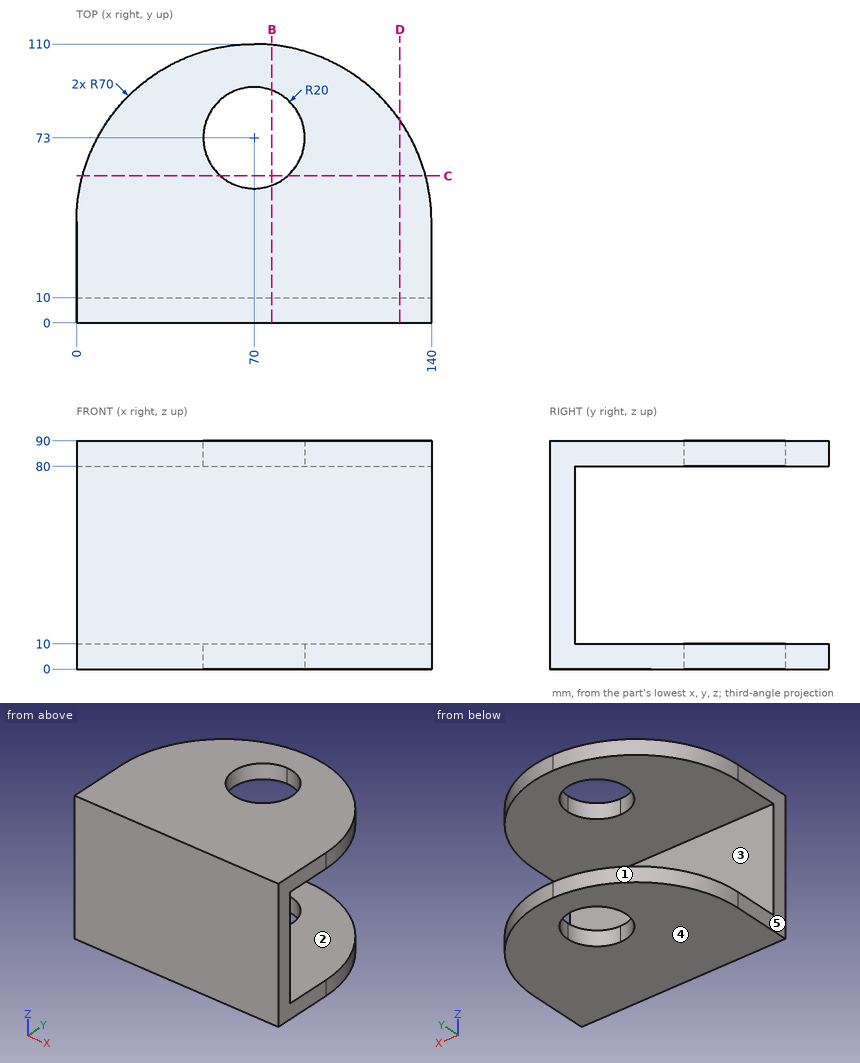
Input: dimensioned drawing with shaded views. Units: mm. Origin: part minimum x, y, z. A direction names the side the tool comes from. Give positions to 0.01 mm unless a question says otherwise; leave off trailing zeros. Loops run counter-clockwise (first coordinate to the right, second up) from the corner with the lowest first, then second, coordinate; pieces in that order, holes last. Notation, with made-up numbers: M -28.75,69.25 L 10.25,69.25 A27 ccw 10.25,97.25 Z; hole C 25,33 d3. An arc over 180 degrees is marked long. Put each result on its own line as item: value.
1) Mould query, pull axis Z, two halves, no side actions, for the marked faces 3, 4 and 5. Classes: released by +Z, released by -Z, zero draft, split by the parting line, or undercut.
Computed values:
face 3: undercut
face 4: released by -Z
face 5: zero draft
2) Reachability of the marked faces 1 and 2 from +Z, -Z, +X, -X, +Y, -Y: full face, straight path, thin tool, end or side. Return the list, or none.
Computed values:
face 1: +Z, -Z, -X, +Y
face 2: +X, -X, +Y
3) First-contact query: P1, Ø12, axis at y = 61, z = 17.5, coming from the -X side; P2, Ø10, axis at x = 104, z = 75.5, coming from the +Y side; P3, Ø21, axis at x = 46, z = 46.5, coming from the +Y side. Flat tips, straight axial feed; report the tip coordinate or a pass-through.
Computed values:
P1: passes through
P2: stops at y = 102.35
P3: stops at y = 10
4) Material intervals for L1, parallel to Z at x = 51.5, y = 60.5; L2, parallel to Y at x = 114, z = 17; L3, parallel to Y at x = 68.5, z = 8, sorted ascending. Write a range as from..to.
Computed values:
L1: z = 0..10, 80..90
L2: y = 0..10
L3: y = 0..53.06, 92.94..109.98
5) Cut plane B-B, the plane x = 77. Return the cut outline in (y, z) (3 decimals).
Computed values:
outline: M 0,0 L 54.265,0 L 54.265,10 L 10,10 L 10,80 L 54.265,80 L 54.265,90 L 0,90 Z; M 91.735,0 L 109.649,0 L 109.649,10 L 91.735,10 Z; M 91.735,80 L 109.649,80 L 109.649,90 L 91.735,90 Z
6) Cut plane C-C, the plane y = 58. Return the cut outline in (x, z), plus the area to 3 significant figures.
Computed values:
outline: M 2.35,0 L 56.77,0 L 56.77,10 L 2.35,10 Z; M 2.35,80 L 56.77,80 L 56.77,90 L 2.35,90 Z; M 83.23,0 L 137.65,0 L 137.65,10 L 83.23,10 Z; M 83.23,80 L 137.65,80 L 137.65,90 L 83.23,90 Z
area: 2,180 mm^2
7) Cut plane D-D, the plane x = 127.5. Return the cut outline in (y, z), plus the area to 3 significant figures.
Computed values:
outline: M 0,0 L 79.92,0 L 79.92,10 L 10,10 L 10,80 L 79.92,80 L 79.92,90 L 0,90 Z
area: 2,300 mm^2
